```python
from build123d import *

# Parameters (mm, degrees)
SKETCH1_R           = 62
SKETCH1_R_2         = 5
SKETCH1_R_3         = 43
BOSS_EXTRUDE2_DEPTH = 10
SKETCH2_R           = 42
CUT_EXTRUDE1_DEPTH  = 3


with BuildPart() as part:
    # Sketch1 → Boss-Extrude2 (new body)
    # profile 1 of 2: a face of its own
    with BuildSketch(Plane.XY):
        Circle(SKETCH1_R)
        with Locations((-22.778896304, 47.300865565)):
            Circle(SKETCH1_R_2, mode=Mode.SUBTRACT)
        with Locations((-41.04615283, 32.733214598)):
            Circle(SKETCH1_R_2, mode=Mode.SUBTRACT)
        with Locations((-51.18371539, 11.682349033)):
            Circle(SKETCH1_R_2, mode=Mode.SUBTRACT)
        with Locations((-51.18371539, -11.682349033)):
            Circle(SKETCH1_R_2, mode=Mode.SUBTRACT)
        with Locations((-41.04615283, -32.733214598)):
            Circle(SKETCH1_R_2, mode=Mode.SUBTRACT)
        with Locations((-22.778896304, -47.300865565)):
            Circle(SKETCH1_R_2, mode=Mode.SUBTRACT)
        with Locations((0, -52.5)):
            Circle(SKETCH1_R_2, mode=Mode.SUBTRACT)
        with Locations((22.778896304, -47.300865565)):
            Circle(SKETCH1_R_2, mode=Mode.SUBTRACT)
        with Locations((41.04615283, -32.733214598)):
            Circle(SKETCH1_R_2, mode=Mode.SUBTRACT)
        with Locations((51.18371539, -11.682349033)):
            Circle(SKETCH1_R_2, mode=Mode.SUBTRACT)
        with Locations((51.18371539, 11.682349033)):
            Circle(SKETCH1_R_2, mode=Mode.SUBTRACT)
        with Locations((41.04615283, 32.733214598)):
            Circle(SKETCH1_R_2, mode=Mode.SUBTRACT)
        with Locations((22.778896304, 47.300865565)):
            Circle(SKETCH1_R_2, mode=Mode.SUBTRACT)
        with Locations((0, 52.5)):
            Circle(SKETCH1_R_2, mode=Mode.SUBTRACT)
        Circle(SKETCH1_R_3, mode=Mode.SUBTRACT)
    # profile 2 of 2: a face of its own
    with BuildSketch(Plane.XY):
        Circle(SKETCH1_R_3)
    extrude(amount=BOSS_EXTRUDE2_DEPTH)

    # Sketch2 → Cut-Extrude1 (cut)
    with BuildSketch(Plane.XY.offset(10)):
        Circle(SKETCH2_R)
    extrude(amount=-CUT_EXTRUDE1_DEPTH, mode=Mode.SUBTRACT)

    # Sketch5 → Revolve1 (revolve)
    with BuildSketch(Plane(origin=(0, 0, 0), x_dir=(1, 0, 0), z_dir=(0, 1, 0))):
        Polygon((0, -6.870835564), (-19, -6.870835564), (-17.437166401, -15.734105341), (-13.81978154, -15.734105341), (-15.206288158, -7.870835564), (0, -7.870835564), align=None)
    revolve(axis=Axis((0, 0, 0), (0, 0, 1)))


solid = part.part
```
The listing builds one solid part. Answer for the finished solid, in the listing's coordinates (mm). A direction names the side the tool comes from. Give positions to 0.01 mm unless a question says otherwise; leave off trailing zeros. Write each loop counter-clockwise with the first axis right and the second up, starting at its lowest first coordinate (ties: lowest second). Pieces come first, ordered by that corner, then holes. Notation, with made-up numbers: (20.5, 87) -> (64.5, 87) arc R5 cw to (64.5, 94) -> close; hole circle Ø9 at (47, 59.25). An arc over 180 degrees is marked (long way). Write item = value, one per line. Start each with the question number.
1) Determine the mould class of faces 4 (the face through (45.665, 30.818, 4.93)), 5 (the face through (12.9, -40.5, 10)), 6 (the face through (21.69, 42.42, 4.93)) for opening direction X: +X half, -X half, draft (parallel to the pull), parting line (faces both ways), or undercut.
2) The part is cut by section B-B, the plane z = 5.25. Count the separate pieces of the cut face and the enclosed holes in it, and give its area (3 significant figures).
3) Which of the six approach directions +Z, -Z, +X, -X, +Y, -Y give full straight-line access (tool end or side, diameter ignored) to faces 1 (the face through (18, -9, 7)), 2 (the face through (17.784, -47.081, 4.93)), 3 (the face through (3.048, 13.726, 14.369))?
4) The part is cut by section D-D, the plane x = 0. Determine the outline of the cut face in (y, z), and give its area (3 significant figures).
5) Each of these flat-tipped pins is pushed along its axis until it touches: pin 1 (8 mm diameter, centred on x = -21.5, z = 11, fed in from -Y); pin 2 (13 mm diameter, centred on x = -51.18, y = 11.68, fed in from +Z); pin 3 (2 mm diameter, centred on y = -18, z = 2, fed in from -X); pin 4 (6 mm diameter, centred on x = 51.18, y = 11.68, fed in from +Z). Where does it stop, or does it pass through?
6) The part is cut by section A-A, the plane x = -22. Determine the outline of the cut face in (y, z).
7) Straight lines are drawn through the part: line 1 along Y through (x, z) = (0, 4.5); line 2 along Y through (x, z) = (-42.5, 7.25); line 3 along X through (y, z) = (-14.5, 5.25). For each, find the intervals that lie inside material, in ascending order.
8) The part is cut by section C-C, the plane y = 0. Determine the outline of the cut face in (x, z), and give its area (3 significant figures).
Solutions:
q1.face_4 = undercut
q1.face_5 = draft
q1.face_6 = undercut
q2.separate_pieces = 1
q2.enclosed_holes = 14
q2.area = 11,000 mm²
q3.face_1 = +Z
q3.face_2 = +Z, -Z
q3.face_3 = none
q4.outline = (-62, 0) -> (-57.5, 0) -> (-57.5, 10) -> (-62, 10) -> close; (-47.5, 0) -> (47.5, 0) -> (47.5, 10) -> (42, 10) -> (42, 7) -> (18.98, 7) -> (17.44, 15.73) -> (13.82, 15.73) -> (15.21, 7.87) -> (-15.21, 7.87) -> (-13.82, 15.73) -> (-17.44, 15.73) -> (-18.98, 7) -> (-42, 7) -> (-42, 10) -> (-47.5, 10) -> close; (57.5, 0) -> (62, 0) -> (62, 10) -> (57.5, 10) -> close
q4.area = 878 mm²
q5.pin_1 = -59.44
q5.pin_2 = 10
q5.pin_3 = -59.62
q5.pin_4 = through
q6.outline = (-57.97, 0) -> (-52.24, 0) -> (-52.24, 10) -> (-57.97, 10) -> close; (-42.36, 0) -> (42.36, 0) -> (42.36, 10) -> (35.78, 10) -> (35.78, 7) -> (-35.78, 7) -> (-35.78, 10) -> (-42.36, 10) -> close; (52.24, 0) -> (57.97, 0) -> (57.97, 10) -> (52.24, 10) -> close
q7.line_1 = -62 to -57.5, -47.5 to 47.5, 57.5 to 62
q7.line_2 = -45.14 to -37.52, -27.95 to 27.95, 37.52 to 45.14
q7.line_3 = -60.28 to -55.31, -47.05 to 47.05, 55.31 to 60.28
q8.outline = (-62, 0) -> (62, 0) -> (62, 10) -> (42, 10) -> (42, 7) -> (18.98, 7) -> (17.44, 15.73) -> (13.82, 15.73) -> (15.21, 7.87) -> (-15.21, 7.87) -> (-13.82, 15.73) -> (-17.44, 15.73) -> (-18.98, 7) -> (-42, 7) -> (-42, 10) -> (-62, 10) -> close
q8.area = 1,080 mm²
